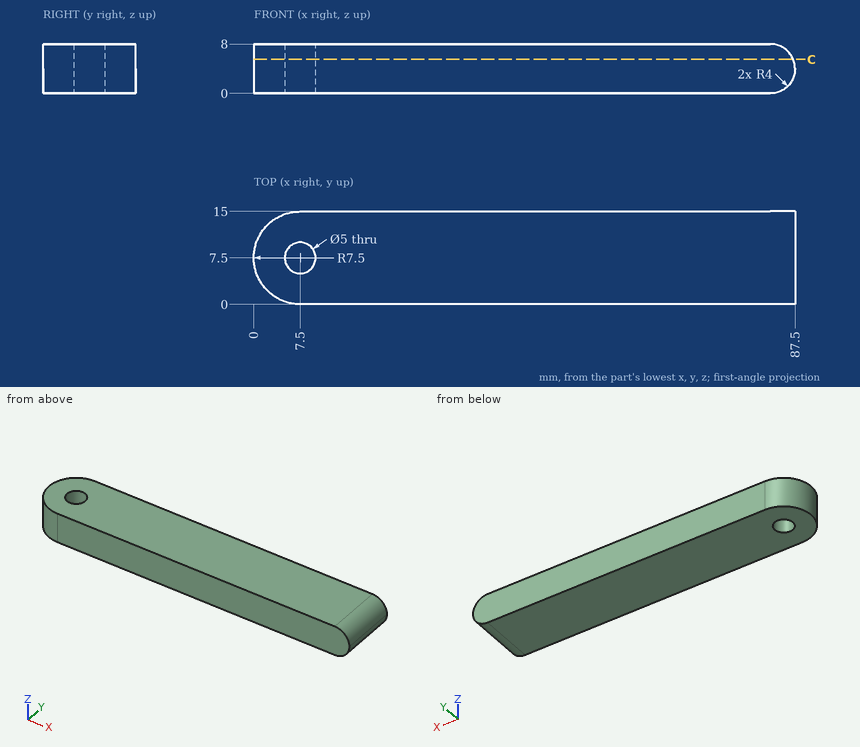
Check sheet for the drawn part. Datum: minimum x, y, z corner. Units: mm. Round coordinates to 2 decimals unless told otherwise and drop trailing zeros. Order: outer loops, then holes, each group sorted by start corner. A loop starts at its lowest first (then second) coordinate and runs counter-clockwise, first axis right, second up. Notation, with made-up numbers: (-16.75, -18.5) -> (34.25, -18.5) arc R20 ccw to (34.25, -6.5) -> close; hole circle Ø4 at (8.25, 27.25). An arc over 180 degrees is marked (long way). Return JSON: item names as keys, results as strings. Group by question number.
Q1. Section check C-C, the plane z = 5.5. Record the boundary of the cut face in (x, y), plus the area to 3 significant figures.
Q2. Material ranges on probe 1 along Y at (x, z) = (7.5, 4.5); probe 2 along X at (y, z) = (7.25, 7); probe 3 along X at (y, z) = (8.75, 0.75) (1 decimal), recorded low to high. Write a range as from..to.
Q3. Gauge pin test, flat ends, axial feed: pin 1 (3 mm diameter, centred on y = 13.5, z = 5, fed in from -X); pin 2 (3 mm diameter, centred on y = 10.5, z = 5, fed in from -X); pin 3 (2 mm diameter, centred on x = 72, z = 4.5, fed in from -Y); pin 4 (3 mm diameter, centred on y = 2.5, z = 3.5, fed in from -X). Record the tip position at first contact, or that the pin passes through.
Numbers:
{
 "1": {"outline": "(7.5, 0) -> (87.21, 0) -> (87.21, 15) -> (7.5, 15) arc R7.5 ccw to start; hole circle Ø5 at (7.5, 7.5)", "area": "1,260 mm^2"},
 "2": {"probe 1": "0..5, 10..15", "probe 2": "0..5.01, 9.99..86.15", "probe 3": "0.1..5.3, 9.7..85.8"},
 "3": {"pin 1": "x = 1.5", "pin 2": "x = 0.15", "pin 3": "y = 0", "pin 4": "x = 0.87"}
}
